Can you work these out from the model? Positions are in its coordinate system, mm. Face numbers are marked on the shaded views. A direction names the side the tool comes from. Give positions to 0.01 mm unless a question says otherwise; leave off trailing zeros. Order: outer loops, then holes, each group sorted by start corner. A loop starts at its lowest first (then second) coordinate and runs counter-clockwise, first axis right, second up.
```python
from build123d import *

# Parameters (mm, degrees)
SKETCH1_W           = 38.1
SKETCH1_H           = 20.32
BOSS_EXTRUDE1_DEPTH = 3.175
SKETCH4_W           = 6.35
SKETCH4_H           = 3.556
CUT_EXTRUDE1_DEPTH  = 3.175
SKETCH5_W           = 3.175
SKETCH5_H           = 8.128
CUT_EXTRUDE2_DEPTH  = 3.175
SKETCH6_W           = 12.7
SKETCH6_H           = 3.175
CUT_EXTRUDE3_DEPTH  = 3.175


with BuildPart() as part:
    # Sketch1 → Boss-Extrude1 (new body)
    with BuildSketch(Plane(origin=(0, 0, 0), x_dir=(1, 0, 0), z_dir=(0, 1, 0))):
        with Locations((19.05, -10.16)):
            Rectangle(SKETCH1_W, SKETCH1_H)
    extrude(amount=BOSS_EXTRUDE1_DEPTH)

    # Sketch4 → Cut-Extrude1 (cut)
    with BuildSketch(Plane(origin=(0, 3.175, 0), x_dir=(1, 0, 0), z_dir=(0, 1, 0))):
        with Locations((31.75, -10.16)):
            Rectangle(SKETCH4_W, SKETCH4_H)
        Polygon((38.1, -15.24), (38.1, -5.08), (34.925, -5.08), (34.925, -8.382), (34.925, -11.938), (34.925, -15.24), align=None)
    extrude(amount=-CUT_EXTRUDE1_DEPTH, mode=Mode.SUBTRACT)

    # Sketch5 → Cut-Extrude2 (cut)
    with BuildSketch(Plane(origin=(0, 3.175, 0), x_dir=(1, 0, 0), z_dir=(0, 1, 0))):
        with Locations((30.95625, -10.16)):
            Rectangle(SKETCH5_W, SKETCH5_H)
    extrude(amount=-CUT_EXTRUDE2_DEPTH, mode=Mode.SUBTRACT)

    # Sketch6 → Cut-Extrude3 (cut)
    with BuildSketch(Plane(origin=(0, 3.175, 0), x_dir=(1, 0, 0), z_dir=(0, 1, 0))):
        with Locations((18.415, -17.4625)):
            Rectangle(SKETCH6_W, SKETCH6_H)
    extrude(amount=-CUT_EXTRUDE3_DEPTH, mode=Mode.SUBTRACT)


solid = part.part
```
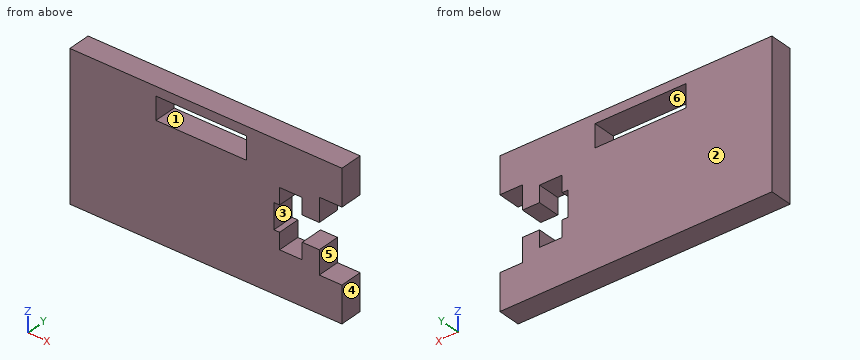
1) Suppose I cut it at D-D (z = 10.5). Please give me the cut outline in (x, y) (3 decimals), and give its area (3 significant figures).
2) Which directions (+Z, -Z, +X, -X, +Y, -Y) give clear straight access to the entire face, cutting with the end or side of a thin tool? Please do the marked faces 4, 5 and 6.
3) If I drill on line 1 (Z direction, x = 34, y = 2); line 2 (Z direction, x = 14, y = 2.95) (3 decimals); line 3 (X direction, y = 2.85, z = 13) (3 decimals), over which ranges is the centre line in solid material (lowest first)?
4) Suppose I cut it at C-C (z = 18.5). Please give me the cut outline in (x, y) (3 decimals).
5) Suppose I cut it at A-A (x = 33). Please give me the cut outline in (y, z) (3 decimals).
6) Suppose I cut it at B-B (y = 1.1). Please give me the cut outline in (x, z) (3 decimals).
7) I'm going to push a flat-ended pin straight in: pin 1 Ø1.8 at (y, z) = (2, 7.5) entering from +X (3 decimals). Where does the tip first touch, or does it pass through?
8) We'd pull the mould along X, two halves only. Please class the marked faces 1, 2 and 3: +X half, -X half, draft (parallel to the pull), parting line (faces both ways), or undercut.
Results:
1. outline: (0, 0) - (28.575, 0) - (28.575, 3.175) - (0, 3.175) - close
1. area: 90.7 mm2
2. face 4: +Z, -Z, +X, +Y, -Y
2. face 5: +X, +Y, -Y
2. face 6: +Y, -Y
3. line 1: z = 0 to 8.38, 11.94 to 20.32
3. line 2: z = 0 to 15.875, 19.05 to 20.32
3. line 3: x = 0 to 29.369, 32.544 to 34.925
4. outline: (0, 0) - (12.065, 0) - (12.065, 3.175) - (0, 3.175) - close; (24.765, 0) - (38.1, 0) - (38.1, 3.175) - (24.765, 3.175) - close
5. outline: (0, 0) - (3.175, 0) - (3.175, 8.382) - (0, 8.382) - close; (0, 11.938) - (3.175, 11.938) - (3.175, 20.32) - (0, 20.32) - close
6. outline: (0, 0) - (38.1, 0) - (38.1, 5.08) - (34.925, 5.08) - (34.925, 8.382) - (32.544, 8.382) - (32.544, 6.096) - (29.369, 6.096) - (29.369, 8.382) - (28.575, 8.382) - (28.575, 11.938) - (29.369, 11.938) - (29.369, 14.224) - (32.544, 14.224) - (32.544, 11.938) - (34.925, 11.938) - (34.925, 15.24) - (38.1, 15.24) - (38.1, 20.32) - (0, 20.32) - close; hole (12.065, 15.875) - (24.765, 15.875) - (24.765, 19.05) - (12.065, 19.05) - close
7. pin 1: stops at x = 34.925
8. face 1: undercut
8. face 2: draft
8. face 3: +X half
